Could you check a few things on this model? Use its own coordinates, in mm. A direction names the side the tool comes from. Coordinates: 2 decimals unless noted, no trailing zeros. Loops run counter-clockwise (first coordinate to the right, second up) from the corner with the lowest first, then second, coordinate; pieces in that order, holes last. Notation, with made-up numbers: (84, 9) -> (98, 9) arc R31 cw to (98, 36) -> close; hole circle Ø3 at (5.5, -8). An arc over 180 degrees is marked (long way). One line per question, with ' | ' between items. Start each with the question number.
(1) Which directions (+Z, -Z, +X, -X, +Y, -Y) give clear straight access to the entire face, cutting with the end or side of a thin tool? Please do faces 1 (the face through (0, 0, 0)), 2 (the face through (-66.701, 0.626, -1.987)).
(2) If we mould it in two halves opening along X, with no side actions, what happens to faces 3 (the face through (-58.79, 0.08, 1.73)), 4 (the face through (-74.4, 0, 0)), 5 (the face through (-31.129, 0.626, -1.987))? For each: pulls with the +X half, pulls with the -X half, needs draft (parallel to the pull), parting line crosses it, or undercut.
(3) I'm going to push flat-ended pins straight in: pin 1 Ø3 at (x, y) = (-54, 0.5) entering from -Z; pin 2 Ø5 at (y, z) = (-1, -3.5) entering from +X; pin 3 Ø3 at (y, z) = (0.5, 3.5) entering from -X; pin 4 Ø2 at (y, z) = (-3, -1.5) entering from -X. Where does each tip first touch, or does it pass through?
(4) Suppose I cut it at C-C (x = -12.5). Please give me the cut outline in (y, z), plus the area to 3 significant figures.
(5) If I drill on line 1 along Z through (x, y) = (-62, 0.75); line 2 along Y through (x, z) = (-41, 0.25); line 3 along X through (y, z) = (-3.25, 0.25), over which ranges is the centre line in solid material (lowest first)?
(6) Suppose I cut it at D-D (z = -3.25). Please give me the cut outline in (x, y), plus the area to 3 significant figures.
(7) Suppose I cut it at A-A (z = 0). Please give me the cut outline in (x, y).
```python
from build123d import *

# Parameters (mm, degrees)
SKETCH1_R           = 4.99999
SKETCH1_R_2         = 2.182749
SKETCH1_R_3         = 2.0828
SKETCH1_R_4         = 1.932813
SKETCH1_R_5         = 1.732788
BOSS_EXTRUDE2_DEPTH = 4.99999
SKETCH1_5_R         = 2.0828
BOSS_EXTRUDE3_DEPTH = 57.999884
BOSS_EXTRUDE4_START = -57.999884
SKETCH1_6_R         = 1.932813
BOSS_EXTRUDE4_DEPTH = 0.199898
BOSS_EXTRUDE5_START = -58.199782
SKETCH1_7_R         = 1.732788
BOSS_EXTRUDE5_DEPTH = 1.199896
BOSS_EXTRUDE6_START = -59.399678
SKETCH1_8_R         = 2.0828
BOSS_EXTRUDE6_DEPTH = 14.99997
CHAMFER1_SIZE       = 0.2032
CHAMFER2_SIZE       = 0.1905


with BuildPart() as part:
    # Sketch1 → Boss-Extrude2 (new body)
    # profile 1 of 5: a face of its own
    with BuildSketch(Plane(origin=(0, 0, 0), x_dir=(0, 0, -1), z_dir=(1, 0, 0))):
        Circle(SKETCH1_R)
        Circle(SKETCH1_R_2, mode=Mode.SUBTRACT)
    # profile 2 of 5: a face of its own
    with BuildSketch(Plane(origin=(0, 0, 0), x_dir=(0, 0, -1), z_dir=(1, 0, 0))):
        Circle(SKETCH1_R_2)
        Circle(SKETCH1_R_3, mode=Mode.SUBTRACT)
    # profile 3 of 5: a face of its own
    with BuildSketch(Plane(origin=(0, 0, 0), x_dir=(0, 0, -1), z_dir=(1, 0, 0))):
        Circle(SKETCH1_R_3)
        Circle(SKETCH1_R_4, mode=Mode.SUBTRACT)
    # profile 4 of 5: a face of its own
    with BuildSketch(Plane(origin=(0, 0, 0), x_dir=(0, 0, -1), z_dir=(1, 0, 0))):
        Circle(SKETCH1_R_4)
        Circle(SKETCH1_R_5, mode=Mode.SUBTRACT)
    # profile 5 of 5: a face of its own
    with BuildSketch(Plane(origin=(0, 0, 0), x_dir=(0, 0, -1), z_dir=(1, 0, 0))):
        Circle(SKETCH1_R_5)
    extrude(amount=-BOSS_EXTRUDE2_DEPTH)

    # Sketch1<5> → Boss-Extrude3 (add)
    with BuildSketch(Plane(origin=(0, 0, 0), x_dir=(0, 0, -1), z_dir=(1, 0, 0))):
        Circle(SKETCH1_5_R)
    extrude(amount=-BOSS_EXTRUDE3_DEPTH)

    # Sketch1<6> → Boss-Extrude4 (add)
    with BuildSketch(Plane(origin=(0, 0, 0), x_dir=(0, 0, -1), z_dir=(1, 0, 0)).offset(BOSS_EXTRUDE4_START)):
        Circle(SKETCH1_6_R)
    extrude(amount=-BOSS_EXTRUDE4_DEPTH)

    # Sketch1<7> → Boss-Extrude5 (add)
    with BuildSketch(Plane(origin=(0, 0, 0), x_dir=(0, 0, -1), z_dir=(1, 0, 0)).offset(BOSS_EXTRUDE5_START)):
        Circle(SKETCH1_7_R)
    extrude(amount=-BOSS_EXTRUDE5_DEPTH)

    # Sketch1<8> → Boss-Extrude6 (add)
    with BuildSketch(Plane(origin=(0, 0, 0), x_dir=(0, 0, -1), z_dir=(1, 0, 0)).offset(BOSS_EXTRUDE6_START)):
        Circle(SKETCH1_8_R)
    extrude(amount=-BOSS_EXTRUDE6_DEPTH)

    # Chamfer1
    # the kernel refuses this chamfer: 0.2032 mm, written as the material it takes off along each edge
    with BuildSketch(Plane(origin=(-58.199782, 0, 0), x_dir=(0, 0, -1), z_dir=(0, -1, 0))) as chamfer1_piece_1_section:
        Polygon((1.932813 - CHAMFER1_SIZE, 0), (1.932813, CHAMFER1_SIZE), (1.932813, 0), align=None)
    chamfer1_piece_1 = revolve(axis=Axis((-58.199782, 0, 0), (1, 0, 0)), mode=Mode.PRIVATE)
    chamfer1_piece_1 = chamfer1_piece_1 - Plane(origin=(-58.102785298, 0, 0), x_dir=(0, 0, -1), z_dir=(1, 0, 0)) * Cylinder(1.732788, 8, mode=Mode.PRIVATE)
    chamfer1_piece_1 = split(chamfer1_piece_1, bisect_by=Plane(origin=(-57.999884, 0, 1.835689298), z_dir=(-1, 0, 0)), keep=Keep.TOP, mode=Mode.PRIVATE)
    add(chamfer1_piece_1, mode=Mode.SUBTRACT)

    # Chamfer2
    chamfer2_edges = [part.edges().sort_by_distance(p)[0] for p in [
        (-74.399648, 0, 2.0828),
    ]]
    chamfer(chamfer2_edges, length=CHAMFER2_SIZE)


solid = part.part
```
Checks:
1) face 1: +Z, -Z, +X, +Y, -Y | face 2: -X
2) face 3: undercut | face 4: pulls with the -X half | face 5: needs draft
3) pin 1: stops at z = -2.08 | pin 2: stops at x = 0 | pin 3: stops at x = -74.26 | pin 4: stops at x = -5
4) outline: circle Ø4.17 at (0, 0) | area: 13.6 mm^2
5) line 1: z = -1.94 to 1.94 | line 2: y = -2.07 to 2.07 | line 3: x = -5 to 0
6) outline: (-5, -3.8) -> (0, -3.8) -> (0, 3.8) -> (-5, 3.8) -> close | area: 38.0 mm^2
7) outline: (-74.4, -1.89) -> (-74.21, -2.08) -> (-59.4, -2.08) -> (-59.4, -1.73) -> (-58.2, -1.73) -> (-58, -1.93) -> (-58, -2.08) -> (-5, -2.08) -> (-5, -5) -> (0, -5) -> (0, 5) -> (-5, 5) -> (-5, 2.08) -> (-58, 2.08) -> (-58, 1.93) -> (-58.2, 1.73) -> (-59.4, 1.73) -> (-59.4, 2.08) -> (-74.21, 2.08) -> (-74.4, 1.89) -> close
